The listing builds one solid part. Answer for the finished solid, in the listing's coordinates (mm). A direction names the side the tool comes from. Coordinates: 2 decimals unless noted, no trailing zeros. Order: outer loops, then holes, each group sorted by start corner. A loop starts at its lowest first (then second) coordinate and runs counter-clockwise, first axis right, second up.
from build123d import *

# Parameters (mm, degrees)
BOSS_EXTRUDE1_DEPTH = 29
SKETCH2_R           = 1.6
CUT_EXTRUDE1_DEPTH  = 88.095866722
SKETCH8_R           = 5
SKETCH8_R_2         = 1.6
CUT_EXTRUDE3_DEPTH  = 107.775184478
CUT_EXTRUDE4_DEPTH  = 107.775184548
FILLET1_R           = 2
FILLET2_R           = 10


with BuildPart() as part:
    # Sketch1 → Boss-Extrude1 (new body)
    with BuildSketch(Plane(origin=(0, 0, 0), x_dir=(1, 0, 0), z_dir=(0, 1, 0))):
        Polygon((0, 0), (0, 45), (68.7, 45), (68.7, 0), (63.7, 0), (63.7, 40), (5, 40), (5, 0), align=None)
    extrude(amount=BOSS_EXTRUDE1_DEPTH)

    # Sketch2 → Cut-Extrude1 (cut, through all)
    with BuildSketch(Plane(origin=(68.7, 0, 0), x_dir=(0, 0, -1), z_dir=(1, 0, 0))):
        with Locations((13, 14.5)):
            Circle(SKETCH2_R)
    extrude(amount=-CUT_EXTRUDE1_DEPTH, mode=Mode.SUBTRACT)

    # Loft2: read off the stored shape, not the designer's step
    # Loft2: loft between two sections, ruled curve by curve
    loft2_from = [
        Edge.make_bspline([(58.7830687, 7.499869108, -75), (59.236789371, 8.574717733, -75), (59.594121179, 9.715673973, -75), (60.075863556, 12.071270035, -75), (60.2, 13.285510166, -75), (60.2, 15.714489834, -75), (60.075863556, 16.928729965, -75), (59.594121179, 19.284326027, -75), (59.236789371, 20.425282267, -75), (58.7830687, 21.500130892, -75)], [0, 0, 0, 0, 0.25, 0.25, 0.5, 0.5, 0.75, 0.75, 1, 1, 1, 1], 3),
        Edge.make_bspline([(58.7830687, 21.500130892, -75), (58.245644387, 22.773270556, -75), (57.518678604, 24.085542636, -75), (56.075347645, 25.993948982, -75), (55.535761632, 26.619337811, -75), (54.335762543, 27.820816595, -75), (53.675268026, 28.396824058, -75), (52.237826073, 29.468150951, -75), (51.460832799, 29.963342143, -75), (49.805218581, 30.841316492, -75), (48.926615313, 31.223945338, -75), (47.093581696, 31.849079498, -75), (46.13924648, 32.091442444, -75), (44.189865052, 32.41694581, -75), (43.194978913, 32.5, -75), (41.205021087, 32.5, -75), (40.210134948, 32.41694581, -75), (38.26075352, 32.091442444, -75), (37.306418304, 31.849079498, -75), (35.473384687, 31.223945338, -75), (34.594781419, 30.841316492, -75), (32.939167201, 29.963342143, -75), (32.162173927, 29.468150951, -75), (30.724731974, 28.396824058, -75), (30.064237457, 27.820816595, -75), (28.864238368, 26.619337811, -75), (28.324652355, 25.993948982, -75), (26.881321396, 24.085542636, -75), (26.154355613, 22.773270556, -75), (25.6169313, 21.500130892, -75)], [0, 0, 0, 0, 0.125, 0.125, 0.1875, 0.1875, 0.25, 0.25, 0.3125, 0.3125, 0.375, 0.375, 0.4375, 0.4375, 0.5, 0.5, 0.5625, 0.5625, 0.625, 0.625, 0.6875, 0.6875, 0.75, 0.75, 0.8125, 0.8125, 0.875, 0.875, 1, 1, 1, 1], 3),
        Edge.make_bspline([(25.6169313, 7.499869108, -75), (26.154355613, 6.226729444, -75), (26.881321396, 4.914457364, -75), (28.324652355, 3.006051018, -75), (28.864238368, 2.380662189, -75), (30.064237457, 1.179183405, -75), (30.724731974, 0.603175942, -75), (32.162173927, -0.468150951, -75), (32.939167201, -0.963342143, -75), (34.594781419, -1.841316492, -75), (35.473384687, -2.223945338, -75), (37.306418304, -2.849079498, -75), (38.26075352, -3.091442444, -75), (40.210134948, -3.41694581, -75), (41.205021087, -3.5, -75), (43.194978913, -3.5, -75), (44.189865052, -3.41694581, -75), (46.13924648, -3.091442444, -75), (47.093581696, -2.849079498, -75), (48.926615313, -2.223945338, -75), (49.805218581, -1.841316492, -75), (51.460832799, -0.963342143, -75), (52.237826073, -0.468150951, -75), (53.675268026, 0.603175942, -75), (54.335762543, 1.179183405, -75), (55.535761632, 2.380662189, -75), (56.075347645, 3.006051018, -75), (57.518678604, 4.914457364, -75), (58.245644387, 6.226729444, -75), (58.7830687, 7.499869108, -75)], [0, 0, 0, 0, 0.125, 0.125, 0.1875, 0.1875, 0.25, 0.25, 0.3125, 0.3125, 0.375, 0.375, 0.4375, 0.4375, 0.5, 0.5, 0.5625, 0.5625, 0.625, 0.625, 0.6875, 0.6875, 0.75, 0.75, 0.8125, 0.8125, 0.875, 0.875, 1, 1, 1, 1], 3),
        Edge.make_bspline([(25.6169313, 21.500130892, -75), (25.163210629, 20.425282267, -75), (24.805878821, 19.284326027, -75), (24.324136444, 16.928729965, -75), (24.2, 15.714489834, -75), (24.2, 13.285510166, -75), (24.324136444, 12.071270035, -75), (24.805878821, 9.715673973, -75), (25.163210629, 8.574717733, -75), (25.6169313, 7.499869108, -75)], [0, 0, 0, 0, 0.25, 0.25, 0.5, 0.5, 0.75, 0.75, 1, 1, 1, 1], 3),
    ]
    loft2_to = [
        Edge.make_bspline([(68.7, 0, -45), (68.7, 2.416666667, -45), (68.7, 4.833333333, -45), (68.7, 9.666666667, -45), (68.7, 12.083333333, -45), (68.7, 16.916666667, -45), (68.7, 19.333333333, -45), (68.7, 24.166666667, -45), (68.7, 26.583333333, -45), (68.7, 29, -45)], [0, 0, 0, 0, 0.25, 0.25, 0.5, 0.5, 0.75, 0.75, 1, 1, 1, 1], 3),
        Edge.make_bspline([(68.7, 29, -45), (65.8375, 29, -45), (62.975, 29, -45), (58.68125, 29, -45), (57.25, 29, -45), (54.3875, 29, -45), (52.95625, 29, -45), (50.09375, 29, -45), (48.6625, 29, -45), (45.8, 29, -45), (44.36875, 29, -45), (41.50625, 29, -45), (40.075, 29, -45), (37.2125, 29, -45), (35.78125, 29, -45), (32.91875, 29, -45), (31.4875, 29, -45), (28.625, 29, -45), (27.19375, 29, -45), (24.33125, 29, -45), (22.9, 29, -45), (20.0375, 29, -45), (18.60625, 29, -45), (15.74375, 29, -45), (14.3125, 29, -45), (11.45, 29, -45), (10.01875, 29, -45), (5.725, 29, -45), (2.8625, 29, -45), (0, 29, -45)], [0, 0, 0, 0, 0.125, 0.125, 0.1875, 0.1875, 0.25, 0.25, 0.3125, 0.3125, 0.375, 0.375, 0.4375, 0.4375, 0.5, 0.5, 0.5625, 0.5625, 0.625, 0.625, 0.6875, 0.6875, 0.75, 0.75, 0.8125, 0.8125, 0.875, 0.875, 1, 1, 1, 1], 3),
        Edge.make_bspline([(0, 0, -45), (2.8625, 0, -45), (5.725, 0, -45), (10.01875, 0, -45), (11.45, 0, -45), (14.3125, 0, -45), (15.74375, 0, -45), (18.60625, 0, -45), (20.0375, 0, -45), (22.9, 0, -45), (24.33125, 0, -45), (27.19375, 0, -45), (28.625, 0, -45), (31.4875, 0, -45), (32.91875, 0, -45), (35.78125, 0, -45), (37.2125, 0, -45), (40.075, 0, -45), (41.50625, 0, -45), (44.36875, 0, -45), (45.8, 0, -45), (48.6625, 0, -45), (50.09375, 0, -45), (52.95625, 0, -45), (54.3875, 0, -45), (57.25, 0, -45), (58.68125, 0, -45), (62.975, 0, -45), (65.8375, 0, -45), (68.7, 0, -45)], [0, 0, 0, 0, 0.125, 0.125, 0.1875, 0.1875, 0.25, 0.25, 0.3125, 0.3125, 0.375, 0.375, 0.4375, 0.4375, 0.5, 0.5, 0.5625, 0.5625, 0.625, 0.625, 0.6875, 0.6875, 0.75, 0.75, 0.8125, 0.8125, 0.875, 0.875, 1, 1, 1, 1], 3),
        Edge.make_bspline([(0, 29, -45), (0, 26.583333333, -45), (0, 24.166666667, -45), (0, 19.333333333, -45), (0, 16.916666667, -45), (0, 12.083333333, -45), (0, 9.666666667, -45), (0, 4.833333333, -45), (0, 2.416666667, -45), (0, 0, -45)], [0, 0, 0, 0, 0.25, 0.25, 0.5, 0.5, 0.75, 0.75, 1, 1, 1, 1], 3),
    ]
    loft2 = Solid(Shell([*[Face.make_surface_from_curves(loft2_from[k], loft2_to[k]) for k in range(4)], Face(Wire(loft2_from)), Face(Wire(loft2_to))]))
    add(loft2)

    # Sketch8 → Cut-Extrude3 (cut, through all)
    with BuildSketch(Plane(origin=(0, 0, -75), x_dir=(-1, 0, 0), z_dir=(0, 0, -1))):
        with Locations((-42.2, 14.5)):
            Circle(SKETCH8_R)
        with Locations((-42.2, 24)):
            Circle(SKETCH8_R_2)
        with Locations((-29.7, 14.5)):
            Circle(SKETCH8_R_2)
        with Locations((-42.2, 5)):
            Circle(SKETCH8_R_2)
        with Locations((-54.7, 14.5)):
            Circle(SKETCH8_R_2)
    extrude(amount=-CUT_EXTRUDE3_DEPTH, mode=Mode.SUBTRACT)

    # Sketch9 → Cut-Extrude4 (cut, through all)
    with BuildSketch(Plane(origin=(68.7, 0, 0), x_dir=(0, 0, -1), z_dir=(1, 0, 0))):
        Polygon((0, 13), (25, 0), (0, 0), align=None)
        Polygon((0, 16), (25, 29), (0, 29), align=None)
    extrude(amount=-CUT_EXTRUDE4_DEPTH, mode=Mode.SUBTRACT)

    # Fillet1
    fillet1_edges = [part.edges().sort_by_distance(p)[0] for p in [
        (2.5, 16, 0),
        (66.2, 16, 0),
        (66.2, 0, -25),
        (2.5, 0, -25),
        (66.2, 29, -25),
        (2.5, 29, -25),
        (2.5, 13, 0),
        (66.2, 13, 0),
    ]]
    fillet(fillet1_edges, radius=FILLET1_R)

    # Fillet2
    fillet2_edges = [part.edges().sort_by_distance(p)[0] for p in [
        (68.7, 14.5, -45),
        (0, 14.5, -45),
    ]]
    fillet(fillet2_edges, radius=FILLET2_R)


solid = part.part
(1) Given pin 1 Ø4 at (x, z) = (25.5, -51.5) entering from +Y; pin 2 Ø15.5 at (x, z) = (50, -38) entering from +Y; pin 3 Ø12 at (y, z) = (12.5, -66) entering from +X, each flat-ended and moving along its own axis, determine where each tip first touches the part or whether it passes through.
(2) The mould has two halves that part along Y. Classify faces 1 (the flat face through (66.235, 22.582, -12.657)), 2 (the cylindrical face through (40.674, 24.481, -57.745)), 3 (the flat face through (2.535, 6.418, -12.657)): pulls with the +Y half, pulls with the -Y half, needs draft (parallel to the pull), parting line crosses it, or undercut.
(3) A tool of negligible diameter and unlimited length cuts with its end or side. For faces 4 (the flat face through (63.7, 14, -24)), 5 (the flat face through (35, 0, -42)), 6 (the flat face through (35, 29, -42)), 7 (the cylindrical face through (37.581, 12.585, -57.745)), 8 (the flat face through (46, 11, -75)), from which of +Z, -Z, +X, -X, +Y, -Y can it reach the whole face along a straight path? Write none if from no direction.
(4) Find section B-B on z = -21. Determine the outline of the cut face in (x, y), then the cut area to 3 significant figures.
(5) Find the intervals of material crossed by probe 1 along X at (y, z) = (3, -35); probe 2 along Z at (x, y) = (36.5, 9); probe 3 along Y at (x, z) = (42.2, -61), in increasing order.
(6) Find section A-A on z = -5.5. Determine the outline of the cut face in (x, y), then the cut area to 3 significant figures.
Resolved:
1. pin 1: stops at y = 29.56
1. pin 2: stops at y = 29.02
1. pin 3: stops at x = 64.43
2. face 1: pulls with the +Y half
2. face 2: undercut
2. face 3: pulls with the -Y half
3. face 4: +Z, +Y, -Y
3. face 5: +Z, +X, -X, -Y
3. face 6: +Z, +X, -X, +Y
3. face 7: +Z, -Z
3. face 8: -Z, +X, -X, +Y, -Y
4. outline: (0, 2.08) - (5, 2.08) - (5, 26.92) - (0, 26.92) - close; (63.7, 2.08) - (68.7, 2.08) - (68.7, 26.92) - (63.7, 26.92) - close
4. area: 248 mm2
5. probe 1: x = 0 to 5, 63.7 to 68.7
5. probe 2: z = -75 to -40
5. probe 3: y = -1.73 to 3.4, 6.6 to 9.5, 19.5 to 22.4, 25.6 to 30.73
6. outline: (0, 10.14) - (5, 10.14) - (5, 18.86) - (0, 18.86) - close; (63.7, 10.14) - (68.7, 10.14) - (68.7, 18.86) - (63.7, 18.86) - close
6. area: 87.2 mm2
